Print and shaded views of the part. All mm, measured from the part's lowest x, y and z. Round coordinates to 2 decimals unless told otherwise and drop trailing zeros. Write each loop counter-clockwise with the first axis right and the second up, starting at its lowest first coordinate (ties: lowest second). Pieces come first, ordered by that corner, then holes. Notation, with made-up numbers: (27.5, -15) - (48.5, -15) arc R30 cw to (48.5, 19) - close; hole circle Ø11 at (32.5, 39.25). An arc over 180 degrees is marked (long way). Put each result on its own line as item: value. Start each with the question number.
Item 1: Cut at B-B (z = 2.6). Count the separate pieces of the cut face and the enclosed holes in it, and give its area (3 significant figures).
Item 2: Cut at A-A (x = 10). Give the cut face in (y, z), and give its area (3 significant figures).
Item 3: Drill centre lines: line 1 (Y direction, x = 10, z = 1.35); line 2 (Y direction, x = 27, z = 4.55); line 3 (X direction, y = 26.5, z = 2.1). Where is each one in solid material? Low to high. Write a range as from..to.
Item 4: Pin check, flat tip, straight feed: pin 1 Ø3 at (x, y) = (40.085, 63.97) entering from +Z. Stop position of the tip, or through.
Item 5: Cut at C-C (y = 90). Give the cut face in (x, z).
Item 6: Cut at D-D (y = 59). Give the cut face in (x, z).
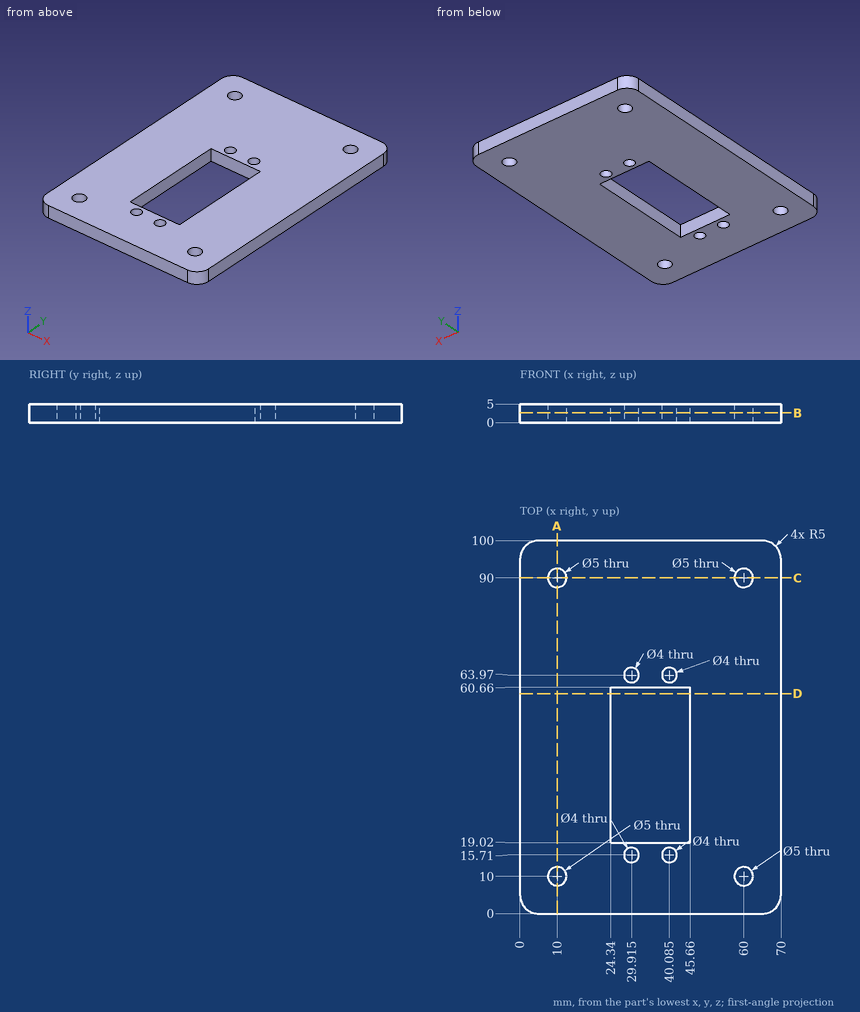
Output values:
1. separate pieces: 1
1. enclosed holes: 9
1. area: 5,960 mm2
2. outline: (0, 0) - (7.5, 0) - (7.5, 5) - (0, 5) - close; (12.5, 0) - (87.5, 0) - (87.5, 5) - (12.5, 5) - close; (92.5, 0) - (100, 0) - (100, 5) - (92.5, 5) - close
2. area: 450 mm2
3. line 1: 0..7.5, 12.5..87.5, 92.5..100
3. line 2: 0..19.02, 60.66..100
3. line 3: 0..24.34, 45.66..70
4. pin 1: through
5. outline: (0, 0) - (7.5, 0) - (7.5, 5) - (0, 5) - close; (12.5, 0) - (57.5, 0) - (57.5, 5) - (12.5, 5) - close; (62.5, 0) - (70, 0) - (70, 5) - (62.5, 5) - close
6. outline: (0, 0) - (24.34, 0) - (24.34, 5) - (0, 5) - close; (45.66, 0) - (70, 0) - (70, 5) - (45.66, 5) - close
